Job drawing, mm, ordinate dimensions from the low corner. One solid piece. A direction names the side the tool comes from. Give positions to 0.01 mm unless a question says otherwise; leave off trailing zeros. Loops run counter-clockwise (first coordinate to the right, second up) from the corner with the lowest first, then second, coordinate; pieces in that order, holes last. Notation, with made-up numbers: (55, -34.75) -> (61, -34.75) arc R23 cw to (61, -4.75) -> close; hole circle Ø4 at (39.5, -16). An arc over 180 degrees is marked (long way). Answer as a JSON object with one key per item and string values. Group by question number.
Q1. Wall check: probe 1 along Y at (x, z) = (24.5, 13); probe 2 along Y at (x, z) = (47.5, 46.75); probe 3 along Z at (x, y) = (8, 137). Give the ranges that are in metal, low to high. Write a range as from..to.
Q2. Tool access for the marked faces 1, 2 and 3: list every direction of +Z, -Z, +X, -X, +Y, -Y with a clear straight run to the whole face (end or side of a thin tool).
Q3. Drop flat-ended pins along their axis: pin 1 (5.5 mm diameter, centred on x = 22.5, y = 125, fed in from -Z); pin 2 (10 mm diameter, centred on y = 20, z = 23, fed in from +X). Give the stop position or say it passes through.
Q4. Band-saw the part on B-B, the plane y = 125. Write the cut outline in (x, z).
Q5. Band-saw the part on A-A, the plane x = 63. Write the cut outline in (y, z).
Q6. Two-plate mould, pull along Y, no slides. Class the marked faces 4, 5 and 6: pulls with the +Y half, pulls with the -Y half, needs draft (parallel to the pull), parting line crosses it, or undercut.
Q7. Band-saw the part on D-D, the plane z = 38. Write the cut outline in (x, y), plus the area to 3 significant figures.
Q8. Band-saw the part on C-C, the plane x = 22.5. Write the cut outline in (y, z), plus the area to 3 significant figures.
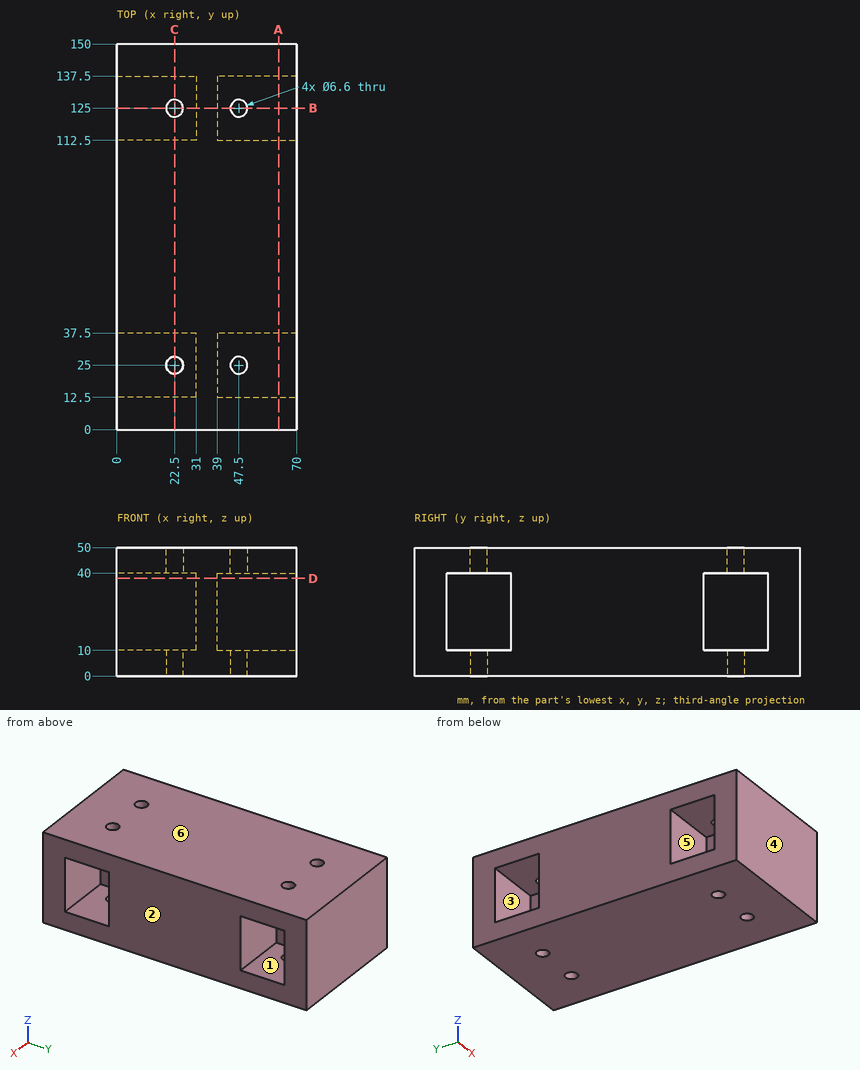
Worked answers:
{
 "1": {"probe 1": "0..12.5, 37.5..112.5, 137.5..150", "probe 2": "0..21.7, 28.3..121.7, 128.3..150", "probe 3": "0..10, 40..50"},
 "2": {"face 1": "+X", "face 2": "+Z, -Z, +X, +Y, -Y", "face 3": "-X"},
 "3": {"pin 1": "through", "pin 2": "x = 39"},
 "4": {"outline": "(0, 0) -> (19.2, 0) -> (19.2, 10) -> (0, 10) -> close; (0, 40) -> (19.2, 40) -> (19.2, 50) -> (0, 50) -> close; (25.8, 0) -> (44.2, 0) -> (44.2, 10) -> (39, 10) -> (39, 40) -> (44.2, 40) -> (44.2, 50) -> (25.8, 50) -> (25.8, 40) -> (31, 40) -> (31, 10) -> (25.8, 10) -> close; (50.8, 0) -> (70, 0) -> (70, 10) -> (50.8, 10) -> close; (50.8, 40) -> (70, 40) -> (70, 50) -> (50.8, 50) -> close"},
 "5": {"outline": "(0, 0) -> (150, 0) -> (150, 50) -> (0, 50) -> close; hole (12.5, 10) -> (37.5, 10) -> (37.5, 40) -> (12.5, 40) -> close; hole (112.5, 10) -> (137.5, 10) -> (137.5, 40) -> (112.5, 40) -> close"},
 "6": {"face 4": "pulls with the -Y half", "face 5": "undercut", "face 6": "needs draft"},
 "7": {"outline": "(0, 0) -> (70, 0) -> (70, 12.5) -> (39, 12.5) -> (39, 37.5) -> (70, 37.5) -> (70, 112.5) -> (39, 112.5) -> (39, 137.5) -> (70, 137.5) -> (70, 150) -> (0, 150) -> (0, 137.5) -> (31, 137.5) -> (31, 112.5) -> (0, 112.5) -> (0, 37.5) -> (31, 37.5) -> (31, 12.5) -> (0, 12.5) -> close", "area": "7,400 mm2"},
 "8": {"outline": "(0, 0) -> (21.7, 0) -> (21.7, 10) -> (12.5, 10) -> (12.5, 40) -> (21.7, 40) -> (21.7, 50) -> (0, 50) -> close; (28.3, 0) -> (121.7, 0) -> (121.7, 10) -> (112.5, 10) -> (112.5, 40) -> (121.7, 40) -> (121.7, 50) -> (28.3, 50) -> (28.3, 40) -> (37.5, 40) -> (37.5, 10) -> (28.3, 10) -> close; (128.3, 0) -> (150, 0) -> (150, 50) -> (128.3, 50) -> (128.3, 40) -> (137.5, 40) -> (137.5, 10) -> (128.3, 10) -> close", "area": "5,740 mm2"}
}
